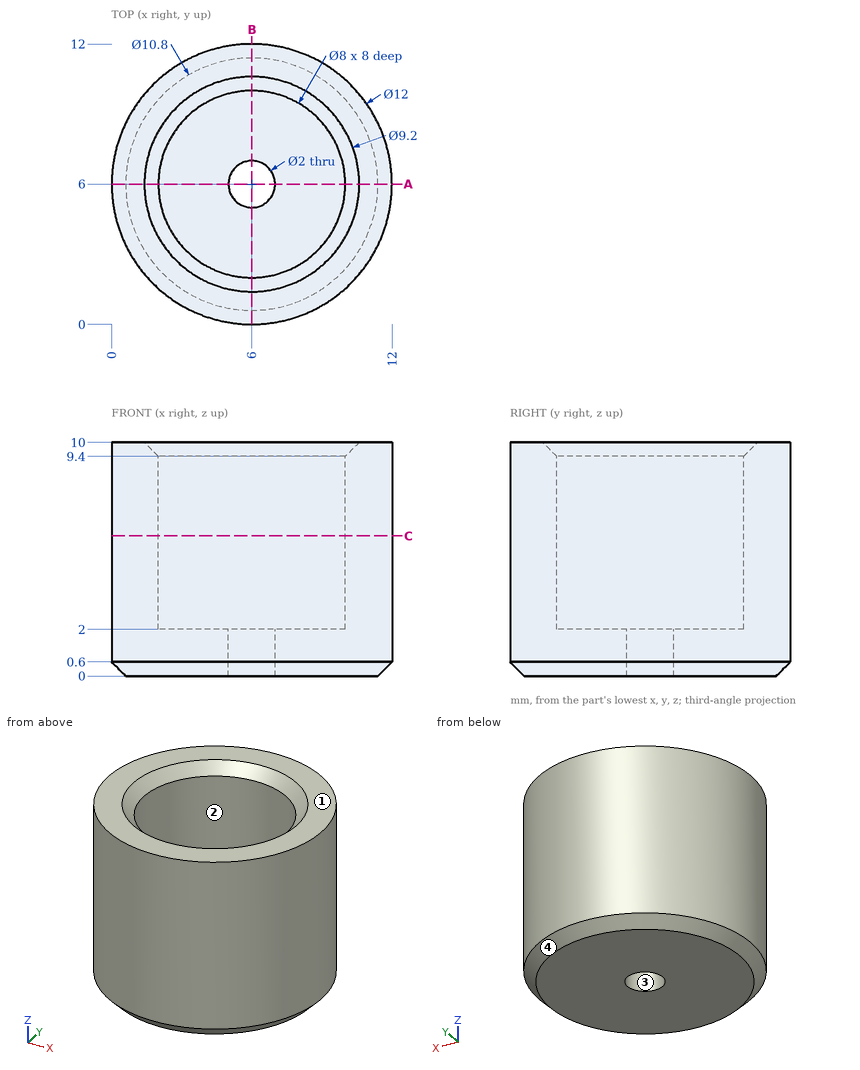
Could you check a few things on this drawing? It's one solid part, dimensions in mm from its lowest x, y, z. Round coordinates to 2 decimals unless told otherwise and drop trailing zeros. Loops run counter-clockwise (first coordinate to the right, second up) from the corner with the lowest first, then second, coordinate; pieces in that order, holes last. Notation, with made-up numbers: (40, -30.5) -> (94, -30.5) arc R12 cw to (94, -11.5) -> close; hole circle Ø2 at (39, 15). An arc over 180 degrees is marked (long way). One line per item, written item: value. Start each with the question number.
1. If we section it at A-A, the plane y = 6: Write out the boundary of the cut face in (x, z), then the cut area to 3 significant figures.
2. If we mould it in two halves opening along Y, with no side actions, what happens to the marked faces 1, 2, 3 and 4? For each: pulls with the +Y half, pulls with the -Y half, needs draft (parallel to the pull), parting line crosses it, or undercut.
3. If I drill on probe 1 along Y at (x, z) = (6, 5.25); probe 2 along Y at (x, z) = (6, 1.55); probe 3 along Z at (x, y) = (8.75, 6), over which ranges is the centre line in solid material (lowest first)?
4. If we section it at C-C, the plane z = 6: Write out the boundary of the cut face in (x, y), then the cut area to 3 significant figures.
5. For pin 1 (5 mm diameter, centred on y = 2, z = 5, fed in from +X); pin 2 (1.8 mm diameter, centred on x = 6, y = 6, fed in from +Z); pin 3 (2 mm diameter, centred on x = 9.5, z = 8.5, fed in from +Y); pin 4 (2 mm diameter, centred on y = 9, z = 5, fed in from -X), each with a flat end and sliding along its axis, tell me the tip position at first contact or that it passes through.
Calculated:
1. outline: (0, 0.6) -> (0.6, 0) -> (5, 0) -> (5, 2) -> (2, 2) -> (2, 9.4) -> (1.4, 10) -> (0, 10) -> close; (7, 0) -> (11.4, 0) -> (12, 0.6) -> (12, 10) -> (10.6, 10) -> (10, 9.4) -> (10, 2) -> (7, 2) -> close
1. area: 51.3 mm²
2. face 1: needs draft
2. face 2: undercut
2. face 3: undercut
2. face 4: parting line crosses it
3. probe 1: y = 0 to 2, 10 to 12
3. probe 2: y = 0 to 5, 7 to 12
3. probe 3: z = 0 to 2
4. outline: circle Ø12 at (6, 6); hole circle Ø8 at (6, 6)
4. area: 62.8 mm²
5. pin 1: stops at x = 11.81
5. pin 2: passes through
5. pin 3: stops at y = 11.45
5. pin 4: stops at x = 0.34
